For this review, take the finished solid that the model builds, in its own axes (mm). Coordinates: 2 decimals unless noted, no trailing zeros. Loops run counter-clockwise (first coordinate to the right, second up) from the corner with the lowest first, then second, coordinate; pieces in that order, holes last. Notation, with made-up numbers: (-2, 49) - (22, 49) arc R14 cw to (22, 74) - close; hole circle Ø11 at (-33.5, 89). An arc over 180 degrees is marked (long way). One line per item, written item: value. Start each with the question number.
1. Take a section at D-D, the plane x = -7. State the section outline as (y, z) points, and give its area (3 significant figures).
2. The part is to be moulded in two halves that separate along Z. For faces 1 (the face through (15, 24.905, 0)), 2 (the face through (-0.96, 0.69, 4.34)), 3 (the face through (0.1, 0.69, 7.48)), 4 (the face through (-14, 20.841, 0)), say which applies: released by +Z, released by -Z, zero draft, split by the parting line, or undercut.
3. Take a section at A-A, the plane x = 0. State the section outline as (y, z) points (3 decimals).
4. To check wall thickness, follow line 1 (Z direction, x = 0, y = 0.45) (3 decimals); line 2 (X direction, y = 23.5, z = 2.25); line 3 (X direction, y = 10.25, z = 3.5). State the ranges of each line that lie inside material, in increasing order. Write a range as from..to.
5. Take a section at B-B, the plane z = -0.75. Count the separate pieces of the cut face and the enclosed holes in it, and give its area (3 significant figures).
6. Take a section at C-C, the plane z = 5.5. State the section outline as (x, y) points, and give its area (3 significant figures).
7. Insertion check: pin 1 (1.5 mm diameter, centred on x = 10.5, z = -1, fed in from -Y); pin 2 (7.5 mm diameter, centred on x = -3.5, z = -0.5, fed in from +Y); pin 3 (6 mm diameter, centred on y = 3.5, z = 4.5, fed in from -X); pin 4 (1.5 mm diameter, centred on y = 14.5, z = -1.5, fed in from -X). Each pin has a flat end and moves straight along its axis. Give the tip position at first contact, or say it passes through.
```python
from build123d import *

# Parameters (mm, degrees)
SKETCH1_R                 = 4.445
BASE_DEPTH                = 1.4097
RADIAL_FLANGE_DEPTH       = 1.905
AXIAL_CUT_OUT_DEPTH       = 4.064
SKETCH6_W                 = 4.064
SKETCH6_H                 = 2.159
RADIAL_CUT_OUT_DEPTH      = 17.5481001
RADIAL_CUT_OUT_DEPTH_BACK = 17.5481001


with BuildPart() as part:
    # Sketch1 → Base (new body)
    with BuildSketch(Plane(origin=(0, 0, 0), x_dir=(1, 0, 0), z_dir=(0, 1, 0))):
        with BuildLine():
            Line((-12.661842678, 4.572), (-5.920447964, 4.572))
            ThreePointArc((-5.920447964, 4.572), (0, 7.4803), (5.920447964, 4.572))
            Line((5.920447964, 4.572), (12.661842678, 4.572))
            ThreePointArc((12.661842678, 4.572), (13.462, 0), (12.661842678, -4.572))
            Line((12.661842678, -4.572), (5.920447964, -4.572))
            ThreePointArc((5.920447964, -4.572), (0, -7.4803), (-5.920447964, -4.572))
            Line((-5.920447964, -4.572), (-12.661842678, -4.572))
            ThreePointArc((-12.661842678, -4.572), (-13.462, 0), (-12.661842678, 4.572))
        make_face()
        Circle(SKETCH1_R, mode=Mode.SUBTRACT)
    extrude(amount=BASE_DEPTH)

    # Sketch3 → Arm loft section 0
    with BuildSketch(Plane(origin=(0, 0, 0), x_dir=(1, 0, 0), z_dir=(0, 1, 0))):
        with BuildLine():
            Line((-12.661842678, -4.572), (-11.163242678, -4.572))
            ThreePointArc((-11.163242678, -4.572), (-12.06321562, 0), (-11.163242678, 4.572))
            Line((-11.163242678, 4.572), (-12.661842678, 4.572))
            ThreePointArc((-12.661842678, 4.572), (-13.462, 0), (-12.661842678, -4.572))
        make_face()
    # Sketch2 → Arm loft section 1
    with BuildSketch(Plane(origin=(0, 24.9047, 0), x_dir=(-1, 0, 0), z_dir=(0, -1, 0))):
        with BuildLine():
            Line((12.244143702, 4.953), (13.874423051, 4.953))
            ThreePointArc((13.874423051, 4.953), (14.732, 0), (13.874423051, -4.953))
            Line((13.874423051, -4.953), (12.244143702, -4.953))
            ThreePointArc((12.244143702, -4.953), (13.208, 0), (12.244143702, 4.953))
        make_face()
    arm_loft = loft()

    # Mirror of arm loft: Arm loft across plane
    add(arm_loft.mirror(Plane(origin=(0, 0, 0), x_dir=(0, 0, 1), z_dir=(1, 0, 0))))

    # Sketch4 → Radial flange (add)
    with BuildSketch(Plane(origin=(0, 24.9047, 0), x_dir=(-1, 0, 0), z_dir=(0, -1, 0))):
        with BuildLine():
            Line((12.437573678, 4.445), (15.939936907, 4.445))
            ThreePointArc((15.939936907, 4.445), (16.5481, 0), (15.939936907, -4.445))
            Line((15.939936907, -4.445), (12.437573678, -4.445))
            ThreePointArc((12.437573678, -4.445), (13.208, 0), (12.437573678, 4.445))
        make_face()
    radial_flange = extrude(amount=RADIAL_FLANGE_DEPTH)

    # Sketch5 → Axial cut-out (cut)
    with BuildSketch(Plane(origin=(0, 24.9047, 0), x_dir=(1, 0, 0), z_dir=(0, 1, 0))):
        with BuildLine():
            Line((-11.247927631, 2.032), (-13.949780823, 2.032))
            ThreePointArc((-13.949780823, 2.032), (-14.097, 0), (-13.949780823, -2.032))
            Line((-13.949780823, -2.032), (-11.247927631, -2.032))
            ThreePointArc((-11.247927631, -2.032), (-11.43, 0), (-11.247927631, 2.032))
        make_face()
    axial_cut_out = extrude(amount=-AXIAL_CUT_OUT_DEPTH, mode=Mode.SUBTRACT)

    # Mirror of radial flange and axial cut-out: Radial flange, Axial cut-out across plane
    add(radial_flange.mirror(Plane(origin=(0, 0, 0), x_dir=(0, 0, 1), z_dir=(1, 0, 0))))
    add(axial_cut_out.mirror(Plane(origin=(0, 0, 0), x_dir=(0, 0, 1), z_dir=(1, 0, 0))), mode=Mode.SUBTRACT)

    # Sketch6 → Radial cut-out (cut, two sides)
    with BuildSketch(Plane(origin=(0, 0, 0), x_dir=(0, 0, -1), z_dir=(1, 0, 0))) as radial_cut_out_sk:
        with Locations((0, 21.9202)):
            Rectangle(SKETCH6_W, SKETCH6_H)
    extrude(amount=RADIAL_CUT_OUT_DEPTH, mode=Mode.SUBTRACT)
    extrude(radial_cut_out_sk.sketch, amount=-RADIAL_CUT_OUT_DEPTH_BACK, mode=Mode.SUBTRACT)


solid = part.part
```
Solutions:
1. outline: (0, -4.57) - (1.41, -4.57) - (1.41, 4.57) - (0, 4.57) - close
1. area: 12.9 mm2
2. face 1: zero draft
2. face 2: undercut
2. face 3: released by +Z
2. face 4: undercut
3. outline: (0, -7.48) - (1.41, -7.48) - (1.41, -4.445) - (0, -4.445) - close; (0, 4.445) - (1.41, 4.445) - (1.41, 7.48) - (0, 7.48) - close
4. line 1: -7.48..-4.445, 4.445..7.48
4. line 2: -16.39..-12.95, 12.95..16.39
4. line 3: -13.54..-12.04, 12.04..13.54
5. separate pieces: 4
5. enclosed holes: 0
5. area: 91.6 mm2
6. outline: (-5.07, 0) - (5.07, 0) - (5.07, 1.41) - (-5.07, 1.41) - close
6. area: 14.3 mm2
7. pin 1: y = 0
7. pin 2: y = 1.41
7. pin 3: x = -13.59
7. pin 4: x = -14.2
